from build123d import *

# Parameters (mm, degrees)
F2_DEPTH = 3
F4_DEPTH = 3


with BuildPart() as f2:
    # F1 (on face) → F2 (new body)
    with BuildSketch(Plane.XZ):
        with BuildLine():
            Line((-1.32116, -5.919504), (-1.32116, -8.640318))
            Line((-1.32116, -8.640318), (-17.590988, -8.640318))
            ThreePointArc((-17.590988, -8.640318), (0, -19.945099), (17.590988, -8.640318))
            Line((17.590988, -8.640318), (1.10096, -8.640318))
            Line((1.10096, -8.640318), (1.10096, -5.919504))
            Line((1.10096, -5.919504), (18.594568, -5.919504))
            ThreePointArc((18.594568, -5.919504), (0, 18.732423), (-18.594568, -5.919504))
            Line((-18.594568, -5.919504), (-18.539109, -5.919504))
            Line((-18.539109, -5.919504), (-1.32116, -5.919504))
        make_face()
    extrude(amount=F2_DEPTH)


with BuildPart() as f4:
    # F3 (on face) → F4 (new body)
    with BuildSketch(Plane.XZ.offset(3)):
        with BuildLine():
            Line((-54.234255, 45.941614), (-67.258485, 45.941614))
            ThreePointArc((-67.258485, 45.941614), (-61.151606, 38.439632), (-52.068938, 35.111145))
            Line((-52.068938, 35.111145), (-52.068938, 40.961377))
            Line((-52.068938, 40.961377), (-48.604425, 40.961377))
            Line((-48.604425, 40.961377), (-48.604425, 35.152427))
            ThreePointArc((-48.604425, 35.152427), (-39.874481, 38.497244), (-33.945055, 45.725081))
            Line((-33.945055, 45.725081), (-46.872169, 45.725081))
            Line((-46.872169, 45.725081), (-46.872169, 49.406122))
            Line((-46.872169, 49.406122), (-32.718549, 49.406122))
            ThreePointArc((-32.718549, 49.406122), (-50.796761, 71.557655), (-68.277544, 48.931689))
            Line((-68.277544, 48.931689), (-54.234255, 48.931689))
            Line((-54.234255, 48.931689), (-54.234255, 45.941614))
        make_face()
    extrude(amount=F4_DEPTH)


solid = f4.part
Can you work these out from the model? Positions are in its coordinate system, mm. A direction names the side the tool comes from. Round coordinates to 2 decimals unless told otherwise and drop trailing zeros. Order: outer loops, then holes, each group sorted by start corner. A loop starts at its lowest first (then second) coordinate and runs counter-clockwise, first axis right, second up. Notation, with made-up numbers: (-13, 42) -> (-9, 42) arc R19 ccw to (-9, 68) -> close; hole circle Ø8 at (41, 38). An arc over 180 degrees is marked (long way). Write each question's results on one line, items separated by ' | '. Start each with the question number.
Item 1: If we section it at C-C, the plane y = -4.3: Write out the boundary of the cut face in (x, z).
Item 2: Thinking about a two-plate mould opening in Z: for faces 1 (the flat face through (-48.604, -4, 38)), 2 (the flat face through (-54.234, -4, 47)), 3 (the cylindrical face through (-61.263, -4.479, 38.52)), which applies, +Z half, -Z half, draft (parallel to the pull), parting line (faces both ways), or undercut?
Item 3: Will these pins go through, and if not, where does the flat tip stop? pin 1 (0.9 mm diameter, centred on y = -5, z = 38.5, fed in from -X); pin 2 (0.9 mm diameter, centred on x = -39.5, y = -4, fed in from -Z); pin 3 (1 mm diameter, centred on x = -37, y = -3.5, fed in from +Z).
Item 4: If we section it at A-A, the plane x = -45: Write out the boundary of the cut face in (y, z), then the cut area to 3 significant figures.
Item 5: If we section it at D-D, the plane z = 69.5: Write out the boundary of the cut face in (x, y), then the cut area to 3 significant figures.
Item 6: Which directions (+Z, -Z, +X, -X, +Y, -Y) give clear straight access to the entire face, cutting with the end or side of a thin tool? Please do faces 4 (the flat face through (-50, -4, 40.961)), 5 (the flat face through (-46.872, -4, 48)), 6 (the flat face through (-61, -4, 48.932)).
Item 7: Please list where these lines run through material, in increasing order: L1, parallel to Z at x = -51, y = -4.45; L2, parallel to Z at x = -58.5, y = -5.35; L3, parallel to X at y = -5.7, z = 47.
Item 8: If we section it at B-B, the plane z = 39.5: Write out the boundary of the cut face in (x, y).
Results:
1) outline: (-68.28, 48.93) -> (-54.23, 48.93) -> (-54.23, 45.94) -> (-67.26, 45.94) arc R18.26 ccw to (-52.07, 35.11) -> (-52.07, 40.96) -> (-48.6, 40.96) -> (-48.6, 35.15) arc R18.26 ccw to (-33.95, 45.73) -> (-46.87, 45.73) -> (-46.87, 49.41) -> (-32.72, 49.41) arc R18.26 ccw (long way) to start
2) face 1: draft | face 2: undercut | face 3: -Z half
3) pin 1: stops at x = -61.83 | pin 2: stops at z = 38.44 | pin 3: stops at z = 66.07
4) outline: (-6, 35.91) -> (-3, 35.91) -> (-3, 45.73) -> (-6, 45.73) -> close; (-6, 49.41) -> (-3, 49.41) -> (-3, 70.69) -> (-6, 70.69) -> close | area: 93.3 mm2
5) outline: (-58.98, -6) -> (-42.13, -6) -> (-42.13, -3) -> (-58.98, -3) -> close | area: 50.5 mm2
6) face 4: -Z, +Y, -Y | face 5: +X, +Y, -Y | face 6: -X, +Y, -Y
7) L1: z = 40.96 to 71.55 | L2: z = 36.87 to 45.94, 48.93 to 69.74 | L3: x = -54.23 to -46.87
8) outline: (-62.5, -6) -> (-52.07, -6) -> (-52.07, -3) -> (-62.5, -3) -> close; (-48.6, -6) -> (-38.61, -6) -> (-38.61, -3) -> (-48.6, -3) -> close
